```python
from build123d import *

# Parameters (mm, degrees)
BOSS_EXTRUDE2_DEPTH = 25
CUT_EXTRUDE4_DEPTH  = 22.5
CUT_EXTRUDE5_DEPTH  = 2
CUT_EXTRUDE6_DEPTH  = 2
CUT_EXTRUDE7_DEPTH  = 2
SKETCH9_R           = 2.4
BOSS_EXTRUDE3_DEPTH = 10


with BuildPart() as part:
    # Sketch1 → Boss-Extrude2 (new body)
    with BuildSketch(Plane(origin=(0, 0, 0), x_dir=(0, 1, 0), z_dir=(0, 0, 1))):
        Polygon((0, 0), (46, 0), (85.837168574, 23), (80.837168574, 31.660254038), (46, 10), (0, 10), (-34.837168574, 31.660254038), (-39.837168574, 23), align=None)
    extrude(amount=BOSS_EXTRUDE2_DEPTH)

    # Sketch5 → Cut-Extrude4 (cut)
    with BuildSketch(Plane.XY.offset(25)):
        Polygon((-24.732050808, -38.837168574), (-29.062177826, -36.337168574), (-7, 0), (-7, 46), (-29.062177826, 82.337168574), (-24.732050808, 84.837168574), (-2, 46), (-2, 0), align=None)
    extrude(amount=-CUT_EXTRUDE4_DEPTH, mode=Mode.SUBTRACT)

    # Sketch6 → Cut-Extrude5 (cut)
    with BuildSketch(Plane.YZ):
        with BuildLine():
            Line((0, 2.5), (10, 2.5))
            ThreePointArc((10, 2.5), (16.477245972, 5.804759365), (17.603057122, 12.988678845))
            Line((17.603057122, 12.988678845), (19.614378278, 15))
            Line((19.614378278, 15), (26.385621722, 15))
            Line((26.385621722, 15), (28.396942878, 12.988678845))
            ThreePointArc((28.396942878, 12.988678845), (29.522754028, 5.804759365), (36, 2.5))
            Line((36, 2.5), (46, 2.5))
            Line((46, 2.5), (46, 25))
            Line((46, 25), (0, 25))
            Line((0, 25), (0, 2.5))
        make_face()
    extrude(amount=-CUT_EXTRUDE5_DEPTH, mode=Mode.SUBTRACT)

    # Sketch7 → Cut-Extrude6 (cut)
    with BuildSketch(Plane(origin=(19.918584287, 11.5, 0), x_dir=(-0.5000000000000007, 0.8660254037844383, 0), z_dir=(0.8660254037844383, 0.5000000000000007, 0))):
        with BuildLine():
            Line((39.837168574, 25), (39.837168574, 2.5))
            Line((39.837168574, 2.5), (49.837168574, 2.5))
            ThreePointArc((49.837168574, 2.5), (56.314414546, 5.804759365), (57.440225697, 12.988678845))
            Line((57.440225697, 12.988678845), (59.451546852, 15))
            Line((59.451546852, 15), (62.837168574, 15))
            Line((62.837168574, 15), (66.222790296, 15))
            Line((66.222790296, 15), (68.234111452, 12.988678845))
            ThreePointArc((68.234111452, 12.988678845), (69.359922602, 5.804759365), (75.837168574, 2.5))
            Line((75.837168574, 2.5), (85.837168574, 2.5))
            Line((85.837168574, 2.5), (85.837168574, 25))
            Line((85.837168574, 25), (39.837168574, 25))
        make_face()
    extrude(amount=-CUT_EXTRUDE6_DEPTH, mode=Mode.SUBTRACT)

    # Sketch8 → Cut-Extrude7 (cut)
    with BuildSketch(Plane(origin=(0, 0, 0), x_dir=(0.5000000000000014, 0.8660254037844378, 0), z_dir=(0.8660254037844378, -0.5000000000000014, 0))):
        with BuildLine():
            Line((-10.424182503, 2.5), (0, 2.5))
            Line((0, 2.5), (0, 25))
            Line((0, 25), (-46, 25))
            Line((-46, 25), (-46, 2.5))
            Line((-46, 2.5), (-35.575817497, 2.5))
            ThreePointArc((-35.575817497, 2.5), (-29.098571525, 5.804759365), (-27.972760375, 12.988678845))
            Line((-27.972760375, 12.988678845), (-25.961439219, 15))
            Line((-25.961439219, 15), (-23, 15))
            Line((-23, 15), (-20.038560781, 15))
            Line((-20.038560781, 15), (-18.027239625, 12.988678845))
            ThreePointArc((-18.027239625, 12.988678845), (-16.901428475, 5.804759365), (-10.424182503, 2.5))
        make_face()
    extrude(amount=-CUT_EXTRUDE7_DEPTH, mode=Mode.SUBTRACT)

    # Sketch9 → Boss-Extrude3 (add)
    with BuildSketch(Plane(origin=(-10, 0, 0), x_dir=(0, -1, 0), z_dir=(-1, 0, 0))):
        with Locations(Location((-23, 12.5, 0), (0, 0, 90))):
            Circle(SKETCH9_R)
        with Locations(Location((-31, 12.5, 0), (0, 0, 90))):
            Circle(SKETCH9_R)
        with Locations(Location((-15, 12.5, 0), (0, 0, 270))):
            Circle(SKETCH9_R)
    extrude(amount=BOSS_EXTRUDE3_DEPTH)


solid = part.part
```
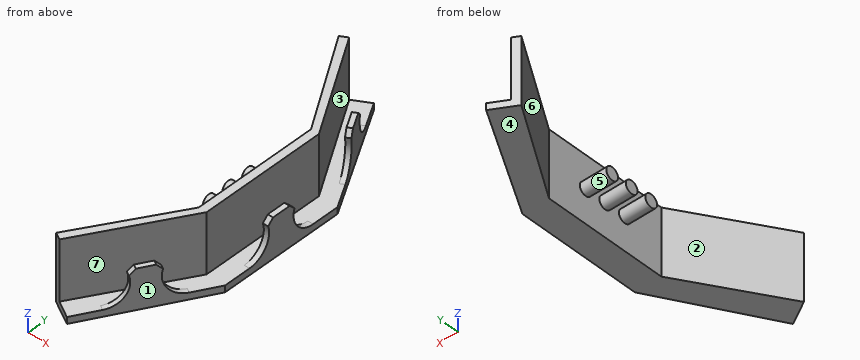
Here's how the part is built. I have some questions about the finished solid (model axes, mm). Face numbers are marked on the shaded views. A direction names the side the tool comes from. Give positions to 0.01 mm unless a question says otherwise; leave off trailing zeros. Loops run counter-clockwise (first coordinate to the right, second up) from the corner with the lowest first, then second, coordinate; pieces in that order, holes last. Notation, with made-up numbers: M 60.25,-9 L 98.25,-9 A15 ccw 98.25,16 Z; hole C 86.5,79.25 d5. An arc over 180 degrees is marked long. Return JSON: item names as keys, results as strings.
Item 1: Imagine slicing it at C-C on z = 11.25. State how many separate pieces and enclosed holes the cut face has, then the cut area to 3 significant figures.
A:
{"separate pieces": "4", "enclosed holes": "0", "area": "549 mm^2"}
Item 2: Imagine slicing it at D-D on y = 40. List the corners of the cut face in (x, z) for me.
A:
{"outline": "M -10,0 L 0,0 L 0,2.5 L -7,2.5 L -7,25 L -10,25 Z"}
Item 3: Thinking about a two-plate mould opening in Y: for the marked faces 1, 2, 3 and 4, which applies, released by +Y, released by -Y, zero draft, split by the parting line, or undercut?
A:
{"face 1": "released by -Y", "face 2": "undercut", "face 3": "undercut", "face 4": "zero draft"}
Item 4: Imagine slicing it at B-B on y = 23. List the corners of the cut face in (x, z) for me.
A:
{"outline": "M -20,10.1 L -10,10.1 L -10,0 L 0,0 L 0,15 L -2,15 L -2,2.5 L -7,2.5 L -7,25 L -10,25 L -10,14.9 L -20,14.9 Z"}
Item 5: Please list where these lines run through material, in increasing order: line 1 (Y direction, x = -21, z = 11.5); line 2 (X direction, y = 38.5, z = 7.25); line 3 (Y direction, x = -25.5, z = 7.25).
A:
{"line 1": "y = -23.06 to -17.69, 63.69 to 69.06", "line 2": "x = -10 to -7", "line 3": "y = -30.47 to -24.93, 70.93 to 76.47"}
Item 6: Imagine slicing it at A-A on z = 20.75. List the corners of the cut face in (x, y) for me, then the cut area to 3 significant figures.
A:
{"outline": "M -31.66,-34.84 L -29.06,-36.34 L -7,0 L -7,46 L -29.06,82.34 L -31.66,80.84 L -10,46 L -10,0 Z", "area": "370 mm^2"}
Item 7: I'm going to push flat-ended pins straight in: pin 1 Ø5.5 at (x, y) = (-11.5, 67) entering from +Z; pin 2 Ø5 at (x, z) = (-7.5, 18.5) entering from +Y; pin 3 Ø10 at (x, z) = (-16.5, 11.5) entering from +Y. Where does each tip first touch, or does it pass through?
A:
{"pin 1": "stops at z = 15", "pin 2": "stops at y = 50.94", "pin 3": "stops at y = 70.97"}
Item 8: On a 3-axis mill with a long thin cutter (end or side, diameter ignored), from which of +Z, -Z, +X, -X, +Y, -Y can I reach the whole of each face in a straight line? I mean the marked faces 5, 6 and 7. Say none if no direction works.
A:
{"face 5": "-X", "face 6": "+Z, -Z, -X", "face 7": "+Z"}
